Read the model definition and answer for the solid it produces. Units are mm, in the model's axes. Give positions to 0.01 mm unless a question says otherwise; leave off trailing zeros. Loops run counter-clockwise (first coordinate to the right, second up) from the corner with the lowest first, then second, coordinate; pieces in that order, holes last.
(1) Each of these flat-tipped pins is pushed along its axis until it touches: P1, Ø3, axis at y = 1, z = -289.5, coming from the -X side; P2, Ø1.5, axis at y = -0.5, z = 102, coming from the +X side; P3, Ø0.6, axis at x = -7.5, z = 33, coming from the -Y side. Where does it stop, or does it pass through?
(2) Straight lines are drawn through the part: probe 1 along X at (y, z) = (-4, 36); probe 2 along Y at (x, z) = (2, -187); probe 3 along Y at (x, z) = (5, -294.5). For each, find the intervals that lie inside material, in ascending order.
(3) Find section A-A, the plane y = -0.25. Write down the section's boundary in (x, z).
Autodesk Inventor part; units mm, degrees
ref_plane "YZ Plane" through (0, 0, 0) normal (1, 0, 0) x (0, 1, 0)
ref_plane "XZ Plane" through (0, 0, 0) normal (0, 1, 0) x (-1, 0, 0)
ref_plane "XY Plane" through (0, 0, 0) normal (0, 0, 1) x (1, 0, 0)
sketch "Esboço1" plane through (0, 0, 0) normal (0, 0, 1) x (1, 0, 0)
  line L0 (7.5, 7.5) -> (-7.5, 7.5) construction
  line L1 (-7.5, 3.1) -> (-7.5, -3.1) construction
  line L2 (-7.5, 7.5) -> (-7.5, 3.1) construction
  line L3 (-7.5, 3.1) -> (-5.5, 3.1) construction
  line L4 (-5.5, 3.1) -> (-5.5, 6.2) construction
  line L5 (-5.5, 6.2) -> (-1.5, 3.1) construction
  line L6 (-1.5, 3.1) -> (-1.5, 0) construction
  line L7 (-1.5, 0) -> (0, 0)
  line L8 (0, 0) -> (0, 7.5)
  arc A0 (-7, 7.5) -> (-7.5, 7) centre (-7, 7) ccw
  line L9 (-7.5, 3.1) -> (-7, 3.1) construction
  line L10 (-7, 3.1) -> (-7, 3.6)
  line L11 (-7, 3.6) -> (-7.5, 3.6)
  line L12 (-7.5, 3.6) -> (-7.5, 3.1) construction
  line L13 (-7.5, 7) -> (-7.5, 3.6)
  line L14 (-7, 7.5) -> (0, 7.5)
  line L15 (-7, 3.1) -> (-5.5, 3.1)
  arc A1 (-5.1775, 5.9501) -> (-5.5, 5.792) centre (-5.3, 5.792) ccw
  line L16 (-5.5, 3.1) -> (-5.5, 5.792)
  arc A2 (-1.5, 2.8549) -> (-1.6937, 3.2501) centre (-2, 2.8549) ccw
  line L17 (-5.1775, 5.9501) -> (-1.6937, 3.2501)
  line L18 (-1.5, 2.8549) -> (-1.5, 0)
  point P0 (-7.5, 0)
  dimension "d0" = 15
  dimension "d1" = 6.2
  dimension "d2" = 7.5
  dimension "d4" = 2
  dimension "d5" = 6
  dimension "d7" = 3.1
  dimension "d10" = 0.5
  dimension "d11" = 0.5
  dimension "d12" = 0.2
  dimension "d13" = 0.5
extrude "Extrusão1" add sketch "Esboço1" along normal mid plane 1000
mirror "Espelhar1" about plane through (0, 0, 0) normal (1, 0, 0) of "Extrusão1"
mirror "Espelhar2" about plane through (0, 0, 0) normal (0, 1, 0) of "Extrusão1", "Espelhar1"
equation "\"d2\" = 0.5 * d0"
properties part number "15×15 2 slots profile_AST01501502" material "Bronze, Cast"
Entries:
1. P1: stops at x = -1.5
1. P2: stops at x = 1.5
1. P3: stops at y = -7.46
2. probe 1: x = -7.5 to -5.5, -2.66 to 2.66, 5.5 to 7.5
2. probe 2: y = -7.5 to -3.49, 3.49 to 7.5
2. probe 3: y = -7.5 to -5.81, 5.81 to 7.5
3. outline: (-1.5, -500) - (1.5, -500) - (1.5, 500) - (-1.5, 500) - close
